Work out the finished part from the listing and answer in its coordinate system (mm). Face numbers are marked on the shaded views. A direction names the side the tool comes from. Round coordinates to 2 decimals unless told otherwise and drop trailing zeros. Order: outer loops, then holes, each group sorted by start corner. A loop starts at its lowest first (then second) coordinate and runs counter-clockwise, first axis right, second up. Notation, with made-up numbers: (-36, 49) -> (-3, 49) arc R32 cw to (-3, 77) -> close; hole circle Ø8 at (-6, -0.75). An arc over 180 degrees is marked (long way). Use a Markdown table: item, result. Add a question column.
Item 1: A cutting plane is placed at A-A, the plane y = -19. Determine the outline of the cut face in (x, z).
Item 2: A cutting plane is placed at C-C, the plane z = -7. Determine the outline of the cut face in (x, y), plus the area to 3 significant figures.
Item 3: A tool of negligible diameter and unlimited length cuts with its end or side. For the marked faces 1 and 2, from which of +Z, -Z, +X, -X, +Y, -Y can it reach the whole face along a straight path? Write none if from no direction.
Item 4: A cutting plane is placed at B-B, the plane x = -2.5. Determine the outline of the cut face in (y, z).
Item 5: Find the intervals of material crossed by L1, parallel to X at y = -0.6, z = 6; L2, parallel to Z at x = -10.75, y = -26.5; L3, parallel to Y at x = -7, z = 3, in increasing order. Write a range as [from, to].
Item 6: Flat-ended cylindrical pins translate along their axes: P1, Ø1, axis at x = 5, z = -19, coming from the -Y side; P2, Ø1.8, axis at x = -4.95, y = -33.95, coming from the +Z side; P3, Ø1.8, axis at x = 0, y = -36, coming from the -Z side. Find the tip coordinate at first contact, or state that the pin passes through.
Item 7: For a pull along Z with two mould halves and no side action, classify the marked faces 3, 4, 5 and 6 as +Z half, -Z half, draft (parallel to the pull), parting line (faces both ways), or undercut.
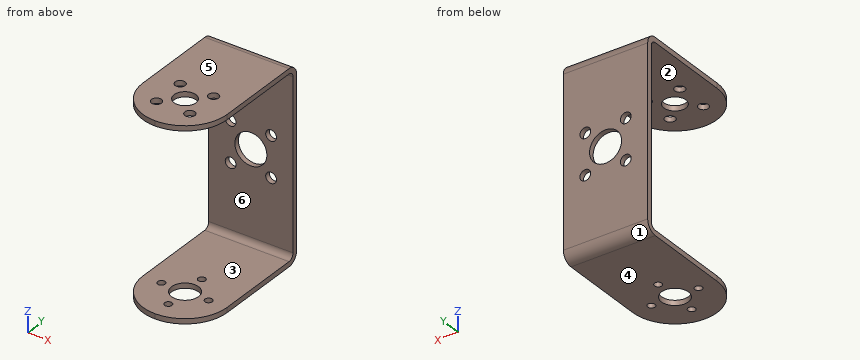
from build123d import *

# Parameters (mm, degrees)
SKETCH1_W                      = 25
SKETCH1_H                      = 53.3
BASE_FLANGE1_DEPTH             = 1.5
EDGE_FLANGE1_STRIP_W           = 9.3
EDGE_FLANGE1_STRIP_H           = 1.5
EDGE_FLANGE1_STRIP_CUT_DEPTH   = 25
EDGE_FLANGE1_STRIP_2_W         = 9.3
EDGE_FLANGE1_STRIP_2_H         = 1.5
EDGE_FLANGE1_STRIP_CUT_2_DEPTH = 25
EDGE_FLANGE1_DEPTH             = 25
EDGE_FLANGE1_BEND_DEPTH        = 25
CUT_EXTRUDE1_REACH             = 73.051
SKETCH12_R                     = 1.5
SKETCH12_R_2                   = 3.25
CUT_EXTRUDE2_REACH             = 73.051
SKETCH13_R                     = 4
SKETCH13_R_2                   = 1.1
FILLET1_R                      = 12.5
SKETCH17_R                     = 1.6
SKETCH17_R_2                   = 4.75
CUT_EXTRUDE3_DEPTH             = 52.680968451


# Sheet-metal steps are written as plain solids
with BuildPart() as part:
    # Base-Flange1: sheet metal written as solids
    # Sketch1 → Base-Flange1 (new body)
    with BuildSketch(Plane(origin=(0, 0, 0), x_dir=(1, 0, 0), z_dir=(0, 1, 0))):
        Rectangle(SKETCH1_W, SKETCH1_H)
    extrude(amount=-BASE_FLANGE1_DEPTH)

    # Edge-Flange1: sheet metal written as solids
    # Edge-Flange1 strip (on a plane across the edge) → Edge-Flange1 strip cut (cut)
    with BuildSketch(Plane(origin=(12.5, -1.5, 26.65), x_dir=(0, 0, -1), z_dir=(-1, 0, 0))):
        with Locations((-3, -0.75)):
            Rectangle(EDGE_FLANGE1_STRIP_W, EDGE_FLANGE1_STRIP_H)
    extrude(amount=EDGE_FLANGE1_STRIP_CUT_DEPTH, mode=Mode.SUBTRACT)

    # Edge-Flange1 strip 2 (on a plane across the edge) → Edge-Flange1 strip cut 2 (cut)
    with BuildSketch(Plane(origin=(-12.5, -1.5, -26.65), x_dir=(0, 0, 1), z_dir=(1, 0, 0))):
        with Locations((-3, -0.75)):
            Rectangle(EDGE_FLANGE1_STRIP_2_W, EDGE_FLANGE1_STRIP_2_H)
    extrude(amount=EDGE_FLANGE1_STRIP_CUT_2_DEPTH, mode=Mode.SUBTRACT)

    # Edge-Flange1 section (on a plane across the edge) → Edge-Flange1 (add)
    with BuildSketch(Plane(origin=(12.5, -1.5, 26.65), x_dir=(0, 0, -1), z_dir=(-1, 0, 0))):
        with BuildLine():
            Line((-1.5, 1.65), (-1.5, 40))
            Line((-1.5, 40), (0, 40))
            Line((0, 40), (0, 1.65))
            ThreePointArc((0, 1.65), (0.483273811, 0.483273811), (1.65, 0))
            Line((1.65, 0), (1.65, -1.5))
            ThreePointArc((1.65, -1.5), (-0.577386361, -0.577386361), (-1.5, 1.65))
        make_face()
    extrude(amount=EDGE_FLANGE1_DEPTH)

    # Edge-Flange1 section 2 (on a plane across the edge) → Edge-Flange1 bend (add)
    with BuildSketch(Plane(origin=(-12.5, -1.5, -26.65), x_dir=(0, 0, 1), z_dir=(1, 0, 0))):
        with BuildLine():
            Line((-1.5, 1.65), (-1.5, 40))
            Line((-1.5, 40), (0, 40))
            Line((0, 40), (0, 1.65))
            ThreePointArc((0, 1.65), (0.483273811, 0.483273811), (1.65, 0))
            Line((1.65, 0), (1.65, -1.5))
            ThreePointArc((1.65, -1.5), (-0.577386361, -0.577386361), (-1.5, 1.65))
        make_face()
    extrude(amount=EDGE_FLANGE1_BEND_DEPTH)

    # Sketch12 → Cut-Extrude1 (cut, up to next)
    with BuildSketch(Plane.XY.offset(28.15), mode=Mode.PRIVATE) as cut_extrude1_sk1:
        with Locations((-4.949747468, -24.050252532)):
            Circle(SKETCH12_R)
    cut_extrude1_tool1 = extrude(cut_extrude1_sk1.sketch, amount=-CUT_EXTRUDE1_REACH, mode=Mode.PRIVATE) & part.part
    # Sketch12 → Cut-Extrude1 (cut, up to next)
    with BuildSketch(Plane.XY.offset(28.15), mode=Mode.PRIVATE) as cut_extrude1_sk2:
        with Locations((4.949747468, -24.050252532)):
            Circle(SKETCH12_R)
    cut_extrude1_tool2 = extrude(cut_extrude1_sk2.sketch, amount=-CUT_EXTRUDE1_REACH, mode=Mode.PRIVATE) & part.part
    # Sketch12 → Cut-Extrude1 (cut, up to next)
    with BuildSketch(Plane.XY.offset(28.15), mode=Mode.PRIVATE) as cut_extrude1_sk3:
        with Locations((-4.949747468, -33.949747468)):
            Circle(SKETCH12_R)
    cut_extrude1_tool3 = extrude(cut_extrude1_sk3.sketch, amount=-CUT_EXTRUDE1_REACH, mode=Mode.PRIVATE) & part.part
    # Sketch12 → Cut-Extrude1 (cut, up to next)
    with BuildSketch(Plane.XY.offset(28.15), mode=Mode.PRIVATE) as cut_extrude1_sk4:
        with Locations((4.949747468, -33.949747468)):
            Circle(SKETCH12_R)
    cut_extrude1_tool4 = extrude(cut_extrude1_sk4.sketch, amount=-CUT_EXTRUDE1_REACH, mode=Mode.PRIVATE) & part.part
    # Sketch12 → Cut-Extrude1 (cut, up to next)
    with BuildSketch(Plane.XY.offset(28.15), mode=Mode.PRIVATE) as cut_extrude1_sk5:
        with Locations((0, -29)):
            Circle(SKETCH12_R_2)
    cut_extrude1_tool5 = extrude(cut_extrude1_sk5.sketch, amount=-CUT_EXTRUDE1_REACH, mode=Mode.PRIVATE) & part.part
    add(cut_extrude1_tool1.solids().sort_by_distance((-4.949747, -24.050253, 28.15))[0], mode=Mode.SUBTRACT)
    add(cut_extrude1_tool2.solids().sort_by_distance((4.949747, -24.050253, 28.15))[0], mode=Mode.SUBTRACT)
    add(cut_extrude1_tool3.solids().sort_by_distance((-4.949747, -33.949747, 28.15))[0], mode=Mode.SUBTRACT)
    add(cut_extrude1_tool4.solids().sort_by_distance((4.949747, -33.949747, 28.15))[0], mode=Mode.SUBTRACT)
    add(cut_extrude1_tool5.solids().sort_by_distance((0, -29, 28.15))[0], mode=Mode.SUBTRACT)

    # Sketch13 → Cut-Extrude2 (cut, up to next)
    with BuildSketch(Plane(origin=(0, 0, -28.15), x_dir=(-1, 0, 0), z_dir=(0, 0, -1)), mode=Mode.PRIVATE) as cut_extrude2_sk1:
        with Locations(Location((0, -29, 0), (0, 0, 90))):
            Circle(SKETCH13_R)
    cut_extrude2_tool1 = extrude(cut_extrude2_sk1.sketch, amount=-CUT_EXTRUDE2_REACH, mode=Mode.PRIVATE) & part.part
    # Sketch13 → Cut-Extrude2 (cut, up to next)
    with BuildSketch(Plane(origin=(0, 0, -28.15), x_dir=(-1, 0, 0), z_dir=(0, 0, -1)), mode=Mode.PRIVATE) as cut_extrude2_sk2:
        with Locations(Location((0, -36, 0), (0, 0, 90))):
            Circle(SKETCH13_R_2)
    cut_extrude2_tool2 = extrude(cut_extrude2_sk2.sketch, amount=-CUT_EXTRUDE2_REACH, mode=Mode.PRIVATE) & part.part
    # Sketch13 → Cut-Extrude2 (cut, up to next)
    with BuildSketch(Plane(origin=(0, 0, -28.15), x_dir=(-1, 0, 0), z_dir=(0, 0, -1)), mode=Mode.PRIVATE) as cut_extrude2_sk3:
        with Locations(Location((-7, -29, 0), (0, 0, 90))):
            Circle(SKETCH13_R_2)
    cut_extrude2_tool3 = extrude(cut_extrude2_sk3.sketch, amount=-CUT_EXTRUDE2_REACH, mode=Mode.PRIVATE) & part.part
    # Sketch13 → Cut-Extrude2 (cut, up to next)
    with BuildSketch(Plane(origin=(0, 0, -28.15), x_dir=(-1, 0, 0), z_dir=(0, 0, -1)), mode=Mode.PRIVATE) as cut_extrude2_sk4:
        with Locations(Location((0, -22, 0), (0, 0, 90))):
            Circle(SKETCH13_R_2)
    cut_extrude2_tool4 = extrude(cut_extrude2_sk4.sketch, amount=-CUT_EXTRUDE2_REACH, mode=Mode.PRIVATE) & part.part
    # Sketch13 → Cut-Extrude2 (cut, up to next)
    with BuildSketch(Plane(origin=(0, 0, -28.15), x_dir=(-1, 0, 0), z_dir=(0, 0, -1)), mode=Mode.PRIVATE) as cut_extrude2_sk5:
        with Locations(Location((7, -29, 0), (0, 0, 90))):
            Circle(SKETCH13_R_2)
    cut_extrude2_tool5 = extrude(cut_extrude2_sk5.sketch, amount=-CUT_EXTRUDE2_REACH, mode=Mode.PRIVATE) & part.part
    add(cut_extrude2_tool1.solids().sort_by_distance((0, -29, -28.15))[0], mode=Mode.SUBTRACT)
    add(cut_extrude2_tool2.solids().sort_by_distance((0, -36, -28.15))[0], mode=Mode.SUBTRACT)
    add(cut_extrude2_tool3.solids().sort_by_distance((7, -29, -28.15))[0], mode=Mode.SUBTRACT)
    add(cut_extrude2_tool4.solids().sort_by_distance((0, -22, -28.15))[0], mode=Mode.SUBTRACT)
    add(cut_extrude2_tool5.solids().sort_by_distance((-7, -29, -28.15))[0], mode=Mode.SUBTRACT)

    # Fillet1
    fillet1_edges = [part.edges().sort_by_distance(p)[0] for p in [
        (12.5, -41.5, 27.4),
        (-12.5, -41.5, 27.4),
        (-12.5, -41.5, -27.4),
        (12.5, -41.5, -27.4),
    ]]
    fillet(fillet1_edges, radius=FILLET1_R - 0.0001)  # a hair under: the kernel refuses the full size

    # Sketch17 → Cut-Extrude3 (cut, through all)
    with BuildSketch(Plane(origin=(0, 0, 0), x_dir=(1, 0, 0), z_dir=(0, 1, 0))):
        with Locations(Location((-6, 6, 0), (0, 0, 270))):
            Circle(SKETCH17_R)
        with Locations(Location((6, 6, 0), (0, 0, 270))):
            Circle(SKETCH17_R)
        with Locations(Location((6, -6, 0), (0, 0, 270))):
            Circle(SKETCH17_R)
        with Locations(Location((-6, -6, 0), (0, 0, 270))):
            Circle(SKETCH17_R)
        with Locations(Location((0, 0, 0), (0, 0, 270))):
            Circle(SKETCH17_R_2)
    extrude(amount=-CUT_EXTRUDE3_DEPTH, mode=Mode.SUBTRACT)


solid = part.part
Reported:
| question | item | result |
|---|---|---|
| 1 | outline | (-12.5, -28.15) -> (12.5, -28.15) -> (12.5, -26.65) -> (-12.5, -26.65) -> close; (-12.5, 26.65) -> (12.5, 26.65) -> (12.5, 28.15) -> (-12.5, 28.15) -> close |
| 2 | outline | (-12.5, -1.5) -> (-7.25, -1.5) -> (-7.25, 0) -> (-12.5, 0) -> close; (-4.75, -1.5) -> (4.75, -1.5) -> (4.75, 0) -> (-4.75, 0) -> close; (7.25, -1.5) -> (12.5, -1.5) -> (12.5, 0) -> (7.25, 0) -> close |
| 2 | area | 30.0 mm² |
| 3 | face 1 | -Z, +X, -X, +Y |
| 3 | face 2 | +X, -X, -Y |
| 4 | outline | (-41.25, -28.15) -> (-32.12, -28.15) -> (-32.12, -26.65) -> (-41.25, -26.65) -> close; (-41.25, 26.65) -> (-31.08, 26.65) -> (-31.08, 28.15) -> (-41.25, 28.15) -> close; (-26.92, 26.65) -> (-3.15, 26.65) arc R1.65 cw to (-1.5, 25) -> (-1.5, 4.04) -> (0, 4.04) -> (0, 25) arc R3.15 ccw to (-3.15, 28.15) -> (-26.92, 28.15) -> close; (-25.88, -28.15) -> (-3.15, -28.15) arc R3.15 ccw to (0, -25) -> (0, -4.04) -> (-1.5, -4.04) -> (-1.5, -25) arc R1.65 cw to (-3.15, -26.65) -> (-25.88, -26.65) -> close |
| 5 | L1 | [-12.5, -7.6], [-4.4, 4.4], [7.6, 12.5] |
| 5 | L2 | [-28.15, -26.65], [26.65, 28.15] |
| 5 | L3 | [-1.5, 0] |
| 6 | P1 | y = -1.5 |
| 6 | P2 | z = -26.65 |
| 6 | P3 | z = 26.65 |
| 7 | face 3 | undercut |
| 7 | face 4 | -Z half |
| 7 | face 5 | +Z half |
| 7 | face 6 | undercut |
